The listing builds one solid part. Answer for the finished solid, in the listing's coordinates (mm). A direction names the side the tool comes from. Round coordinates to 2 decimals unless told otherwise and drop trailing zeros. Order: outer loops, then holes, each group sorted by start corner. A loop starts at its lowest first (then second) coordinate and runs counter-clockwise, first axis right, second up. Notation, with made-up numbers: (60, 38.5) - (97, 38.5) arc R22 ccw to (97, 75.5) - close; hole circle Ø5 at (58.5, 88). An arc over 180 degrees is marked (long way). One line per item, written item: value. Start each with the question number.
1. Section A-A, the plane x = 98.5 is taken. Give the vertices of the cut face in (y, z), then the cut area to 3 significant figures.
2. For a pull along Z with two mould halves and no side action, classify faces 3 (the cylindrical face through (117.966, 3.944, 37.948)), 4 (the cylindrical face through (51.38, 3.94, -39)) as released by +Z, released by -Z, zero draft, split by the parting line, or undercut.
3. Section B-B, the plane x = 33 is taken. Give the vertices of the cut face in (y, z), then the cut area to 3 significant figures.
4. Section C-C, the plane y = 2 is taken. Count the separate pieces of the cut face and the enclosed holes in it, then the cut area to 3 significant figures.
5. A tool of negligible diameter and unlimited length cuts with its end or side. For faces 1 (the flat face through (75, 4, -22.997)), 2 (the cylindrical face through (32.66, 3.94, 39.47)), from which of +Z, -Z, +X, -X, +Y, -Y can it reach the whole face along a straight path? Write none if from no direction.
6. Straight lines are drawn through the part: line 1 (Z direction, x = 125.5, y = 1.5); line 2 (Z direction, x = 129, y = 3.25); line 3 (Z direction, x = 112, y = 0.5). For each, find the intervals that lie inside material, in ascending order.
7. Flat-ended cylindrical pins translate along their axes: P1, Ø2.5, axis at x = 119.5, z = -37.99, coming from the +Y side; P2, Ø1, axis at y = 6, z = -33.5, coming from the -X side. Find the tip coordinate at first contact, or state that the pin passes through.
from build123d import *

# Parameters (mm, degrees)
SKETCH1_R           = 1.5
BOSS_EXTRUDE3_DEPTH = 8


with BuildPart() as part:
    # Sketch1 → Boss-Extrude3 (new body)
    with BuildSketch(Plane(origin=(0, 0, 0), x_dir=(1, 0, 0), z_dir=(0, 1, 0))):
        Polygon((21, 42.996794864), (21, 22.996794864), (130.982222222, 22.996794864), (130.982222222, -23.003205136), (20.982222222, -23.003205136), (20.982222222, -43.003205136), (144.482222222, -43.003205136), (144.482222222, -40.503205136), (144.482222222, 42.996794864), align=None)
        with BuildLine():
            ThreePointArc((133.652222222, -34), (128.132224278, -33.006627887), (133.649820291, -32))
            Line((133.649820291, -32), (135.832222222, -32))
            Line((135.832222222, -32), (135.832222222, -34))
            Line((135.832222222, -34), (133.652222222, -34))
        make_face(mode=Mode.SUBTRACT)
        with BuildLine():
            ThreePointArc((27.482222222, -38.003205136), (24.92156205, -39.063865308), (25.982222222, -36.503205136))
            ThreePointArc((25.982222222, -36.503205136), (27.042882394, -36.942544965), (27.482222222, -38.003205136))
        make_face(mode=Mode.SUBTRACT)
        with Locations((32.982222222, -38.003205136)):
            Circle(SKETCH1_R, mode=Mode.SUBTRACT)
        with Locations((52.475249167, -37.951512162)):
            Circle(SKETCH1_R, mode=Mode.SUBTRACT)
        with Locations((59.475249167, -37.951512162)):
            Circle(SKETCH1_R, mode=Mode.SUBTRACT)
        with Locations((82.343483879, -38.002656399)):
            Circle(SKETCH1_R, mode=Mode.SUBTRACT)
        with Locations((89.343483879, -38.002656399)):
            Circle(SKETCH1_R, mode=Mode.SUBTRACT)
        with Locations((112.464813863, -38.013925916)):
            Circle(SKETCH1_R, mode=Mode.SUBTRACT)
        with Locations((119.464813863, -38.013925916)):
            Circle(SKETCH1_R, mode=Mode.SUBTRACT)
        with Locations((134.24655623, -16.49373389)):
            Circle(SKETCH1_R, mode=Mode.SUBTRACT)
        with Locations((141.24655623, -16.49373389)):
            Circle(SKETCH1_R, mode=Mode.SUBTRACT)
        with Locations((134.24655623, -6.49373389)):
            Circle(SKETCH1_R, mode=Mode.SUBTRACT)
        with Locations((141.24655623, -6.49373389)):
            Circle(SKETCH1_R, mode=Mode.SUBTRACT)
        with BuildLine():
            ThreePointArc((27.5, 27.996794864), (24.939339828, 26.936134692), (26, 29.496794864))
            ThreePointArc((26, 29.496794864), (27.060660172, 29.057455035), (27.5, 27.996794864))
        make_face(mode=Mode.SUBTRACT)
        with Locations((33, 27.996794864)):
            Circle(SKETCH1_R, mode=Mode.SUBTRACT)
        with Locations((52.486589883, 27.989732879)):
            Circle(SKETCH1_R, mode=Mode.SUBTRACT)
        with Locations((26, 37.996794864)):
            Circle(SKETCH1_R, mode=Mode.SUBTRACT)
        with Locations((33, 37.996794864)):
            Circle(SKETCH1_R, mode=Mode.SUBTRACT)
        with Locations((52.486589883, 37.989732879)):
            Circle(SKETCH1_R, mode=Mode.SUBTRACT)
        with Locations((59.486589883, 27.989732879)):
            Circle(SKETCH1_R, mode=Mode.SUBTRACT)
        with Locations((82.502017716, 27.999509045)):
            Circle(SKETCH1_R, mode=Mode.SUBTRACT)
        with Locations((59.486589883, 37.989732879)):
            Circle(SKETCH1_R, mode=Mode.SUBTRACT)
        with Locations((82.502017716, 37.999509045)):
            Circle(SKETCH1_R, mode=Mode.SUBTRACT)
        with Locations((134.199672827, 6.49839835)):
            Circle(SKETCH1_R, mode=Mode.SUBTRACT)
        with Locations((141.199672827, 6.49839835)):
            Circle(SKETCH1_R, mode=Mode.SUBTRACT)
        with Locations((134.199672827, 16.49839835)):
            Circle(SKETCH1_R, mode=Mode.SUBTRACT)
        with Locations((141.199672827, 16.49839835)):
            Circle(SKETCH1_R, mode=Mode.SUBTRACT)
        with Locations((89.502017716, 27.999509045)):
            Circle(SKETCH1_R, mode=Mode.SUBTRACT)
        with Locations((112.502146229, 27.991574488)):
            Circle(SKETCH1_R, mode=Mode.SUBTRACT)
        with Locations((89.502017716, 37.999509045)):
            Circle(SKETCH1_R, mode=Mode.SUBTRACT)
        with Locations((112.502146229, 37.991574488)):
            Circle(SKETCH1_R, mode=Mode.SUBTRACT)
        with Locations((119.502146229, 27.991574488)):
            Circle(SKETCH1_R, mode=Mode.SUBTRACT)
        with Locations((119.502146229, 37.991574488)):
            Circle(SKETCH1_R, mode=Mode.SUBTRACT)
        with BuildLine():
            Line((133.67, 33.996794864), (135.85, 33.996794864))
            Line((135.85, 33.996794864), (135.85, 31.996794864))
            Line((135.85, 31.996794864), (133.67, 31.996794864))
            ThreePointArc((133.67, 31.996794864), (128.114444444, 32.996794864), (133.67, 33.996794864))
        make_face(mode=Mode.SUBTRACT)
        with Locations((89.343483879, -28.002656399)):
            Circle(SKETCH1_R, mode=Mode.SUBTRACT)
        with Locations((112.464813863, -28.013925916)):
            Circle(SKETCH1_R, mode=Mode.SUBTRACT)
        with Locations((119.464813863, -28.013925916)):
            Circle(SKETCH1_R, mode=Mode.SUBTRACT)
        with Locations((52.475249167, -27.951512162)):
            Circle(SKETCH1_R, mode=Mode.SUBTRACT)
        with Locations((59.475249167, -27.951512162)):
            Circle(SKETCH1_R, mode=Mode.SUBTRACT)
        with Locations((25.982222222, -28.003205136)):
            Circle(SKETCH1_R, mode=Mode.SUBTRACT)
        with Locations((32.982222222, -28.003205136)):
            Circle(SKETCH1_R, mode=Mode.SUBTRACT)
        with Locations((82.343483879, -28.002656399)):
            Circle(SKETCH1_R, mode=Mode.SUBTRACT)
    extrude(amount=BOSS_EXTRUDE3_DEPTH)


solid = part.part
Answer list:
1. outline: (0, -43) - (8, -43) - (8, -23) - (0, -23) - close; (0, 23) - (8, 23) - (8, 43) - (0, 43) - close
1. area: 320 mm²
2. face 3: undercut
2. face 4: undercut
3. outline: (0, -43) - (8, -43) - (8, -39.5) - (0, -39.5) - close; (0, -36.5) - (8, -36.5) - (8, -29.5) - (0, -29.5) - close; (0, -26.5) - (8, -26.5) - (8, -23) - (0, -23) - close; (0, 23) - (8, 23) - (8, 26.5) - (0, 26.5) - close; (0, 29.5) - (8, 29.5) - (8, 36.5) - (0, 36.5) - close; (0, 39.5) - (8, 39.5) - (8, 43) - (0, 43) - close
3. area: 224 mm²
4. separate pieces: 1
4. enclosed holes: 42
4. area: 5,220 mm²
5. face 1: -X, +Y, -Y
5. face 2: +Y, -Y
6. line 1: z = -43 to -23, 23 to 43
6. line 2: z = -43 to -35.07, -30.92 to -23, 23 to 30.96, 35.05 to 43
6. line 3: z = -43 to -39.41, -36.58 to -29.41, -26.58 to -23, 23 to 26.59, 29.44 to 36.59, 39.44 to 43
7. P1: passes through
7. P2: stops at x = 21
